CAD build for the part. Positions are in the model's coordinates, mm. Face numbers are marked on the shaded views. Give positions to 0.01 mm unless a question says otherwise; leave off trailing zeros. Loops run counter-clockwise (first coordinate to the right, second up) from the corner with the lowest first, then second, coordinate; pieces in that order, holes last. Notation, with made-up numbers: M 38,-11.75 L 68,-11.75 A18 ccw 68,5.25 Z; hole C 12,4 d10. An arc over 180 degrees is marked long. Answer as CSV lines item,"result".
```python
from build123d import *

# Parameters (mm, degrees)
F1_DEPTH = 25
F2_R     = 0.9
F3_DEPTH = 10
F2_R_2   = 1.55
F4_DEPTH = 24.001
F5_R     = 2


with BuildPart() as f1:
    # F0 (on Front) → F1 (new body)
    with BuildSketch(Plane.XZ):
        with BuildLine():
            Line((-14, -12), (14, -12))
            Line((14, -12), (14, -0.5))
            Line((14, -0.5), (8.119017, -0.5))
            ThreePointArc((8.119017, -0.5), (0.05, 0), (8.119017, 0.5))
            Line((8.119017, 0.5), (14, 0.5))
            Line((14, 0.5), (14, 12))
            Line((14, 12), (-14, 12))
            Line((-14, 12), (-14, -12))
        make_face()
    extrude(amount=F1_DEPTH)

    # F2 (on face) → F3 (cut)
    with BuildSketch(Plane.XY.offset(12)):
        with Locations((-10, -4)):
            Circle(F2_R)
        with Locations((-10, -21)):
            Circle(F2_R)
    extrude(amount=-F3_DEPTH, mode=Mode.SUBTRACT)

    # F2 (on face) → F4 (cut, through all)
    with BuildSketch(Plane.XY.offset(12)):
        with Locations((10, -21)):
            Circle(F2_R_2)
        with Locations((10, -4)):
            Circle(F2_R_2)
    extrude(amount=-F4_DEPTH, mode=Mode.SUBTRACT)

    # F5
    f5_edges = [f1.edges().sort_by_distance(p)[0] for p in [
        (-14, 0, 0),
        (14, -25, -6.25),
        (14, -25, 6.25),
        (14, 0, 6.25),
        (14, 0, -6.25),
        (-14, -25, 0),
    ]]
    fillet(f5_edges, radius=F5_R)


solid = f1.part
```
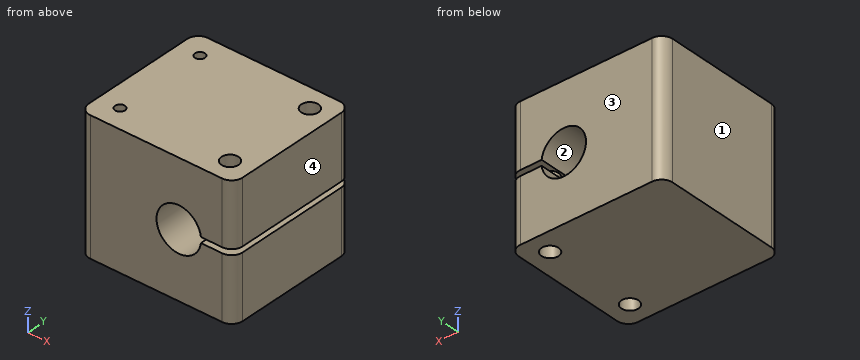
Q1. Cut at D-D (z = -5.75). Write the cut outline in (x, y), and give its area (3 significant figures).
Solution:
outline,"M -14,-23 A2 ccw -12,-25 L 12,-25 A2 ccw 14,-23 L 14,-2 A2 ccw 12,0 L -12,0 A2 ccw -14,-2 Z; hole C 10,-21 d3.1; hole C 10,-4 d3.1"
area,"681 mm²"
Q2. Cut at C-C (y = -21). Write the cut outline in (x, z).
Solution:
outline,"M -14,-12 L 8.45,-12 L 8.45,-0.5 L 8.12,-0.5 A4.05 cw long 8.12,0.5 L 8.45,0.5 L 8.45,12 L -9.1,12 L -9.1,2 L -10.9,2 L -10.9,12 L -14,12 Z; M 11.55,-12 L 14,-12 L 14,-0.5 L 11.55,-0.5 Z; M 11.55,0.5 L 14,0.5 L 14,12 L 11.55,12 Z"
Q3. Mould opens along X. For the marked faces 1, 2, 3 and 4 say: released by +X, released by -X, zero draft, split by the parting line, or undercut.
Solution:
face 1,"released by -X"
face 2,"undercut"
face 3,"zero draft"
face 4,"released by +X"
Q4. Cut at A-A (x = 4.1). Write the cut outline in (y, z), and give its area (4 significant figures).
Solution:
outline,"M -25,-12 L 0,-12 L 0,-4.05 L -25,-4.05 Z; M -25,4.05 L 0,4.05 L 0,12 L -25,12 Z"
area,"397.5 mm²"
Q5. Wall check: line 1 (Y direction, x = 10, z = 3.5); line 2 (Y direction, x = -10, z = 4.25); line 3 (Z direction, x = 12.75, y = -10.25). Give the ranges that are in metal, low to high. Write a range as [from, to].
Solution:
line 1,"y = [-25, -22.55], [-19.45, -5.55], [-2.45, 0]"
line 2,"y = [-25, -21.9], [-20.1, -4.9], [-3.1, 0]"
line 3,"z = [-12, -0.5], [0.5, 12]"
Q6. Cut at B-B (z = 2.75). Write the cut outline in (x, y), and give its area (3 significant figures).
Solution:
outline,"M -14,-23 A2 ccw -12,-25 L 1.13,-25 L 1.13,0 L -12,0 A2 ccw -14,-2 Z; M 7.07,-25 L 12,-25 A2 ccw 14,-23 L 14,-2 A2 ccw 12,0 L 7.07,0 Z; hole C -10,-21 d1.8; hole C -10,-4 d1.8; hole C 10,-21 d3.1; hole C 10,-4 d3.1"
area,"528 mm²"
